Check sheet for the modelled part. Datum: model origin and axes. Units: mm. Round coordinates to 2 decimals unless told otherwise and drop trailing zeros. Order: outer loops, then holes, each group sorted by start corner. A loop starts at its lowest first (then second) coordinate and runs counter-clockwise, first axis right, second up. Notation, with made-up numbers: (-39, 24) -> (6, 24) arc R18 cw to (6, 39) -> close; hole circle Ø9 at (75, 67.5). An arc over 180 degrees is marked (long way). Answer in a Markdown table with one row per item.
```python
from build123d import *

# Parameters (mm, degrees)
ESQUISSE1_W        = 90
ESQUISSE1_H        = 90
ESQUISSE1_R        = 1
ESQUISSE1_R_2      = 0.9
BOSS_EXTRU_2_DEPTH = 5
ESQUISSE2_W        = 10
ESQUISSE2_H        = 5
ESQUISSE2_W_2      = 5
ESQUISSE2_H_2      = 10
CR_NEAUX_DEPTH     = 5


with BuildPart() as part:
    # Esquisse1 → Boss.-Extru.2 (new body)
    with BuildSketch(Plane.XY):
        with Locations((40, 39.6)):
            Rectangle(ESQUISSE1_W, ESQUISSE1_H)
        with Locations((20.816873759, 61.215218426)):
            Circle(ESQUISSE1_R, mode=Mode.SUBTRACT)
        with Locations((68.310891386, 45.405465436)):
            Circle(ESQUISSE1_R, mode=Mode.SUBTRACT)
        with Locations((30.872234855, 12.179316138)):
            Circle(ESQUISSE1_R, mode=Mode.SUBTRACT)
        with Locations((11.611234754, 33.677331021)):
            Circle(ESQUISSE1_R_2, mode=Mode.SUBTRACT)
        with BuildLine():
            Line((49.997987668, 15.058397717), (52.713992085, 11.870640851))
            Line((52.713992085, 11.870640851), (67.902534408, 24.811448374))
            Line((67.902534408, 24.811448374), (64.461892674, 29.40854246))
            ThreePointArc((64.461892674, 29.40854246), (21.335796244, 58.41216357), (49.997987668, 15.058397717))
        make_face(mode=Mode.SUBTRACT)
        Polygon((57.507314904, 9.408845516), (69.87315206, 23.142499017), (74.68907042, 18.806226648), (62.323233265, 5.072573147), align=None, mode=Mode.SUBTRACT)
    extrude(amount=BOSS_EXTRU_2_DEPTH)

    # Esquisse2 → Créneaux - (cut)
    with BuildSketch(Plane(origin=(0, 0, 0), x_dir=(-1, 0, 0), z_dir=(0, 0, -1))):
        with Locations((-75, 74.5)):
            Rectangle(ESQUISSE2_W, ESQUISSE2_H)
        with Locations((-5, 74.5)):
            Rectangle(ESQUISSE2_W, ESQUISSE2_H)
        with Locations((-17.5, 77.1)):
            Rectangle(ESQUISSE2_W, ESQUISSE2_H)
        with Locations((-75, 2.1)):
            Rectangle(ESQUISSE2_W, ESQUISSE2_H)
        with Locations((-5, 2.1)):
            Rectangle(ESQUISSE2_W, ESQUISSE2_H)
        with Locations((-62.5, 77.1)):
            Rectangle(ESQUISSE2_W, ESQUISSE2_H)
        with Locations((-2.5, 17.1)):
            Rectangle(ESQUISSE2_W_2, ESQUISSE2_H_2)
        with Locations((-2.5, 62.1)):
            Rectangle(ESQUISSE2_W_2, ESQUISSE2_H_2)
        with Locations((-17.5, 2.1)):
            Rectangle(ESQUISSE2_W, ESQUISSE2_H)
        with Locations((-50, 2.1)):
            Rectangle(ESQUISSE2_W, ESQUISSE2_H)
        with Locations((-77.5, 62.1)):
            Rectangle(ESQUISSE2_W_2, ESQUISSE2_H_2)
        with Locations((-77.5, 29.6)):
            Rectangle(ESQUISSE2_W_2, ESQUISSE2_H_2)
    extrude(amount=-CR_NEAUX_DEPTH, mode=Mode.SUBTRACT)


solid = part.part
```
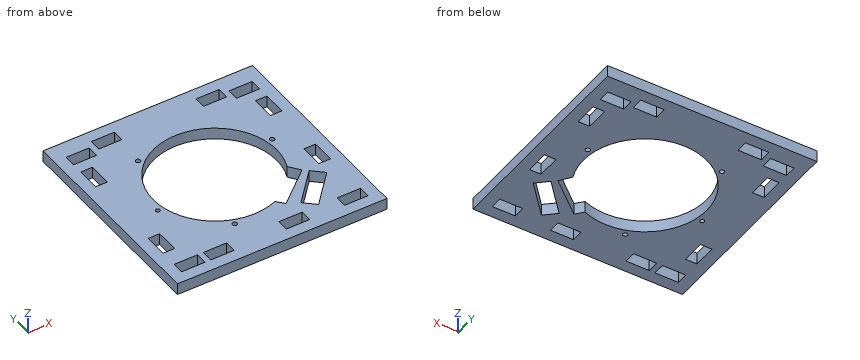
(1) Section check D-D on x = 60. Record the boundary of the cut face in (y, z).
Solutions:
| item | result |
|---|---|
| outline | (-5.4, 0) -> (7.16, 0) -> (7.16, 5) -> (-5.4, 5) -> close; (12.18, 0) -> (18.08, 0) -> (18.08, 5) -> (12.18, 5) -> close; (56.99, 0) -> (74.6, 0) -> (74.6, 5) -> (56.99, 5) -> close; (79.6, 0) -> (84.6, 0) -> (84.6, 5) -> (79.6, 5) -> close |
(2) Section check B-B on y = 39.6. Record the boundary of the cut face in (x, z), plus the area to 3 significant figures.
Solutions:
| item | result |
|---|---|
| outline | (-5, 0) -> (13.5, 0) -> (13.5, 5) -> (-5, 5) -> close; (66.5, 0) -> (85, 0) -> (85, 5) -> (66.5, 5) -> close |
| area | 185 mm^2 |
(3) Depth check by flat-ended pin: pin 1 Ø2.5 at (x, y) = (30.87, 12.18) entering from +Z. Enter the tip coordinate at first touch or a pass-through.
Solutions:
| item | result |
|---|---|
| pin 1 | z = 5 |
(4) Scan lines: probe 1 along X at (y, z) = (79.5, 3.15); probe 2 along Y at (x, z) = (2.5, 0.55); probe 3 along X at (y, z) = (67, 3.2). Record each from-to range of solid material in increasing order. Write a range as from..to.
Solutions:
| item | result |
|---|---|
| probe 1 | -5..12.5, 22.5..57.5, 67.5..85 |
| probe 2 | -5.4..-0.4, 4.6..12.1, 22.1..57.1, 67.1..72, 77..84.6 |
| probe 3 | -5..0, 5..75, 80..85 |
(5) Section check C-C on x = 40. Record the boundary of the cut face in (y, z), plus the area to 3 significant figures.
Solutions:
| item | result |
|---|---|
| outline | (-5.4, 0) -> (13.1, 0) -> (13.1, 5) -> (-5.4, 5) -> close; (66.1, 0) -> (84.6, 0) -> (84.6, 5) -> (66.1, 5) -> close |
| area | 185 mm^2 |
(6) Section check A-A on x = 77. Record the boundary of the cut face in (y, z), plus the area to 3 significant figures.
Solutions:
| item | result |
|---|---|
| outline | (-5.4, 0) -> (-0.4, 0) -> (-0.4, 5) -> (-5.4, 5) -> close; (4.6, 0) -> (24.6, 0) -> (24.6, 5) -> (4.6, 5) -> close; (34.6, 0) -> (57.1, 0) -> (57.1, 5) -> (34.6, 5) -> close; (67.1, 0) -> (72, 0) -> (72, 5) -> (67.1, 5) -> close; (77, 0) -> (84.6, 0) -> (84.6, 5) -> (77, 5) -> close |
| area | 300 mm^2 |
